from build123d import *

# Parameters (mm, degrees)
SKETCH_1_R          = 1.5
EXTRUDE_1_DEPTH     = 3
FILLET_1_R          = 5
SKETCH_2_R          = 1.5
CUT_EXTRUDE_1_DEPTH = 10


with BuildPart() as part:
    # 草圖1 → 填料-伸長1 (new body)
    with BuildSketch(Plane.XY):
        Polygon((15, 120), (160, 120), (160, 0), (15, 0), (0, 60), align=None)
        with Locations((20, 20)):
            Circle(SKETCH_1_R, mode=Mode.SUBTRACT)
        with Locations((20, 100)):
            Circle(SKETCH_1_R, mode=Mode.SUBTRACT)
        with Locations((140, 20)):
            Circle(SKETCH_1_R, mode=Mode.SUBTRACT)
        with Locations((140, 100)):
            Circle(SKETCH_1_R, mode=Mode.SUBTRACT)
    extrude(amount=EXTRUDE_1_DEPTH)

    # 圓角1
    fillet_1_edges = [part.edges().sort_by_distance(p)[0] for p in [
        (160, 0, 1.5),
        (15, 0, 1.5),
        (15, 120, 1.5),
        (160, 120, 1.5),
    ]]
    fillet(fillet_1_edges, radius=FILLET_1_R)

    # 草圖2 → 除料-伸長1 (cut)
    with BuildSketch(Plane.XY.offset(3)):
        with Locations((145.7, 3.38)):
            Circle(SKETCH_2_R)
        with Locations((145.7, 55.38)):
            Circle(SKETCH_2_R)
    extrude(amount=-CUT_EXTRUDE_1_DEPTH, mode=Mode.SUBTRACT)


solid = part.part
Here's how the part is built. I have some questions about the finished solid (model axes, mm). Round coordinates to 2 decimals unless told otherwise and drop trailing zeros. Loops run counter-clockwise (first coordinate to the right, second up) from the corner with the lowest first, then second, coordinate; pieces in that order, holes last. Notation, with made-up numbers: (69, 23.25) - (86, 23.25) arc R15 ccw to (86, 29.25) - close; hole circle Ø9 at (49, 61). An arc over 180 degrees is marked (long way). One line per question, with ' | ' between items. Start each with the question number.
Q1. Will this pin go through, and if not, where does the flat tip stop? pin 1 (1.5 mm diameter, centred on x = 16.5, z = 0.5, fed in from -Y).
Q2. I want a section at A-A (z = 2.2). Write out the boundary of the cut face in (x, y), then the cut area to 3 significant figures.
Q3. I want a section at C-C (y = 107). Write out the boundary of the cut face in (x, z), then the cut area to 3 significant figures.
Q4. I want a section at B-B (y = 80). Write out the boundary of the cut face in (x, z), then the cut area to 3 significant figures.
Q5. Please list where these lines run through material, in increasing order: line 1 (Y direction, x = 140, z = 0.55); line 2 (Y direction, x = 145.7, z = 1.1); line 3 (X direction, y = 19, z = 2.1). Write a range as [from, to].
Response values:
1) pin 1: stops at y = 0.28
2) outline: (0, 60) - (14.05, 3.79) arc R5 ccw to (18.9, 0) - (155, 0) arc R5 ccw to (160, 5) - (160, 115) arc R5 ccw to (155, 120) - (18.9, 120) arc R5 ccw to (14.05, 116.21) - close; hole circle Ø3 at (20, 20); hole circle Ø3 at (20, 100); hole circle Ø3 at (140, 20); hole circle Ø3 at (140, 100); hole circle Ø3 at (145.7, 3.38); hole circle Ø3 at (145.7, 55.38) | area: 18,200 mm²
3) outline: (11.75, 0) - (160, 0) - (160, 3) - (11.75, 3) - close | area: 445 mm²
4) outline: (5, 0) - (160, 0) - (160, 3) - (5, 3) - close | area: 465 mm²
5) line 1: y = [0, 18.5], [21.5, 98.5], [101.5, 120] | line 2: y = [0, 1.88], [4.88, 53.88], [56.88, 120] | line 3: x = [10.25, 18.88], [21.12, 138.88], [141.12, 160]
